Design review of the part built by this model. Coordinates are the model's own, in mm. Face numbers are marked on the shaded views. A direction names the side the tool comes from. Coordinates: 2 decimals unless noted, no trailing zeros. Order: outer loops, then holes, each group sorted by start corner. A loop starts at its lowest first (then second) coordinate and runs counter-clockwise, first axis right, second up. Notation, with made-up numbers: (33.25, -34) -> (68.25, -34) arc R20 ccw to (68.25, -8) -> close; hole circle Ø7 at (10.5, 54). An arc over 180 degrees is marked (long way). Write item = value, one per line.
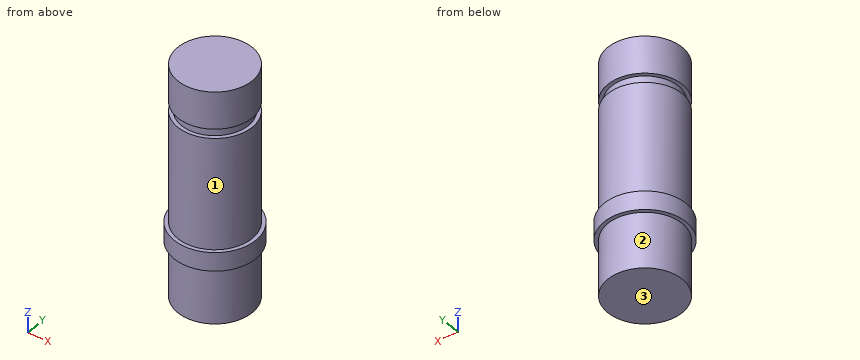
```python
from build123d import *

# Parameters (mm, degrees)
SKETCH_1_R      = 20
EXTRUDE_1_DEPTH = 20
SKETCH_2_R      = 18
EXTRUDE_2_DEPTH = 5
EXTRUDE_START   = 60
SKETCH_3_R      = 20
EXTRUDE_3_DEPTH = 60
SKETCH_4_R      = 22
EXTRUDE_4_DEPTH = 10
EXTRUDE_START_2 = 30
SKETCH_5_R      = 20
EXTRUDE_5_DEPTH = 30


with BuildPart() as part:
    # 草图1 → 凸台-拉伸1 (new body)
    with BuildSketch(Plane.XY):
        Circle(SKETCH_1_R)
    extrude(amount=EXTRUDE_1_DEPTH)

    # 草图2 → 凸台-拉伸2 (add)
    with BuildSketch(Plane(origin=(0, 0, 0), x_dir=(-1, 0, 0), z_dir=(0, 0, -1))):
        Circle(SKETCH_2_R)
    extrude(amount=EXTRUDE_2_DEPTH)

    # 草图3 → 凸台-拉伸3 (add)
    with BuildSketch(Plane(origin=(0, 0, -5), x_dir=(-1, 0, 0), z_dir=(0, 0, -1)).offset(EXTRUDE_START)):
        with Locations(Location((0, 0, 0), (0, 0, 180))):
            Circle(SKETCH_3_R)
    extrude(amount=-EXTRUDE_3_DEPTH)

    # 草图4 → 凸台-拉伸4 (add)
    with BuildSketch(Plane(origin=(0, 0, -65), x_dir=(-1, 0, 0), z_dir=(0, 0, -1))):
        Circle(SKETCH_4_R)
    extrude(amount=EXTRUDE_4_DEPTH)

    # 草图5 → 凸台-拉伸5 (add)
    with BuildSketch(Plane(origin=(0, 0, -75), x_dir=(-1, 0, 0), z_dir=(0, 0, -1)).offset(EXTRUDE_START_2)):
        with Locations(Location((0, 0, 0), (0, 0, 180))):
            Circle(SKETCH_5_R)
    extrude(amount=-EXTRUDE_5_DEPTH)


solid = part.part
```
(1) Insertion check: pin 1 (3 mm diameter, centred on y = -1.5, z = -50.5, fed in from -X); pin 2 (1 mm diameter, centred on x = -11, z = -6.5, fed in from +Y); pin 3 (5 mm diameter, centred on y = -17, z = -60.5, fed in from +X) (3 decimals). Each pin has a flat end and moves straight along its axis. Give the tip position at first contact, or say it passes through.
Report:
pin_1 = -20
pin_2 = 17.02
pin_3 = 13.775
(2) For the marked faces 1, 2 and 3, list the 3-axis set-ups (+Z, -Z, +X, -X, +Y, -Y) from which the entire face can be reached by the end or side of a thin tool; tool diameter is ignored.
Report:
face_1 = +Z
face_2 = -Z
face_3 = -Z, +X, -X, +Y, -Y
(3) We need section C-C (z = -20). Write out the cut boundary in (x, y).
Report:
outline = circle Ø40 at (0, 0)
(4) For L1, parallel to Y at x = 1, z = -45.5; L2, parallel to Z at x = 17.5, y = 10.5; L3, parallel to Y at x = 13.5, z = -12.5, list the stretches that pass through material, from the lowest coordinate up.
Report:
L1 = -19.97 to 19.97
L2 = -75 to -65
L3 = -14.76 to 14.76
(5) We need section B-B (x = 9). Write out the cut boundary in (y, z), and give its area (3 significant figures).
Report:
outline = (-20.07, -75) -> (-17.86, -75) -> (-17.86, -105) -> (17.86, -105) -> (17.86, -75) -> (20.07, -75) -> (20.07, -65) -> (17.86, -65) -> (17.86, -5) -> (15.59, -5) -> (15.59, 0) -> (17.86, 0) -> (17.86, 20) -> (-17.86, 20) -> (-17.86, 0) -> (-15.59, 0) -> (-15.59, -5) -> (-17.86, -5) -> (-17.86, -65) -> (-20.07, -65) -> close
area = 4,490 mm²
(6) We need section A-A (y = 11). Write out the cut boundary in (x, z), and give its area (3 significant figures).
Report:
outline = (-19.05, -75) -> (-16.7, -75) -> (-16.7, -105) -> (16.7, -105) -> (16.7, -75) -> (19.05, -75) -> (19.05, -65) -> (16.7, -65) -> (16.7, -5) -> (14.25, -5) -> (14.25, 0) -> (16.7, 0) -> (16.7, 20) -> (-16.7, 20) -> (-16.7, 0) -> (-14.25, 0) -> (-14.25, -5) -> (-16.7, -5) -> (-16.7, -65) -> (-19.05, -65) -> close
area = 4,200 mm²
